```python
from build123d import *

# Parameters (mm, degrees)
F0_R     = 15
F0_R_2   = 14
F1_DEPTH = 0.85
F4_R     = 14
F3_R     = 5
F6_R     = 3.5
F7_DEPTH = 7


with BuildPart() as f1:
    # F0 (on Front) → F1 (new body)
    with BuildSketch(Plane.XZ):
        Circle(F0_R)
        Circle(F0_R_2, mode=Mode.SUBTRACT)
        Circle(F0_R_2)
    extrude(amount=F1_DEPTH)

    # F4 (on face) → F5 section 0
    with BuildSketch(Plane.XZ.offset(0.85)):
        Circle(F4_R)
    # F3 (on offset) → F5 section 1
    with BuildSketch(Plane.XZ.offset(15.15)):
        Circle(F3_R)
    loft()

    # F6 (on face) → F7 (cut)
    with BuildSketch(Plane.XZ.offset(15.15)):
        Circle(F6_R)
    extrude(amount=-F7_DEPTH, mode=Mode.SUBTRACT)


solid = f1.part
```
Build history of the part. All positions in model axes, mm. A direction names the side the tool comes from. Coordinates: 2 decimals unless noted, no trailing zeros. Order: outer loops, then holes, each group sorted by start corner. A loop starts at its lowest first (then second) coordinate and runs counter-clockwise, first axis right, second up.
Item 1: Drop flat-ended pins along their axis: pin 1 Ø1 at (x, z) = (-4, -5.5) entering from -Y; pin 2 Ø8 at (y, z) = (-8.5, -4.5) entering from -X; pin 3 Ø4 at (x, z) = (8, 4.5) entering from -Y. Give the stop position or say it passes through.
Filled in:
pin 1: stops at y = -13.08
pin 2: stops at x = -11.12
pin 3: stops at y = -11.69
Item 2: Saw through at C-C on y = -3.25. List the corners of the cut face in (x, z).
Filled in:
outline: circle Ø24.98 at (0, 0)
Item 3: Saw through at D-D on y = -12.75. List the corners of the cut face in (x, z).
Filled in:
outline: circle Ø13.02 at (0, 0); hole circle Ø7 at (0, 0)
Item 4: Saw through at A-A on x = 0. List the corners of the cut face in (y, z).
Filled in:
outline: (-15.15, -5) - (-0.85, -14) - (-0.85, -15) - (0, -15) - (0, 15) - (-0.85, 15) - (-0.85, 14) - (-15.15, 5) - (-15.15, 3.5) - (-8.15, 3.5) - (-8.15, -3.5) - (-15.15, -3.5) - close
Item 5: Saw through at B-B on y = -10. List the corners of the cut face in (x, z), then the cut area to 3 significant figures.
Filled in:
outline: circle Ø16.48 at (0, 0); hole circle Ø7 at (0, 0)
area: 175 mm2
Item 6: Tool access for faces 1 (the cylindrical face through (-14.985, -0.419, 0.66)), 2 (the flat face through (0, -8.15, 0)): list every direction of +Z, -Z, +X, -X, +Y, -Y with a clear straight run to the whole face (end or side of a thin tool).
Filled in:
face 1: +Y, -Y
face 2: -Y
Item 7: Drill centre lines: L1, parallel to Z at x = 0, y = -10; L2, parallel to Z at x = -3, y = -13.5; L3, parallel to Y at x = 3.25, z = 1. Where is each one in solid material? Low to high.
Filled in:
L1: z = -8.24 to -3.5, 3.5 to 8.24
L2: z = -5.24 to -1.8, 1.8 to 5.24
L3: y = -8.15 to 0
Item 8: Mould opens along Z. For faces 3 (the cylindrical face through (3.233, -11.699, -1.341)), 4 (the flat face through (2.2, -15.15, -3.3)), 5 (the conical face through (-0.84, -12.87, 6.38)) say: released by +Z, released by -Z, zero draft, split by the parting line, or undercut.
Filled in:
face 3: undercut
face 4: zero draft
face 5: split by the parting line
